from build123d import *

# Parameters (mm, degrees)
CROQUIS1_W              = 29
CROQUIS1_H              = 16
CROQUIS1_R              = 1.5
SALIENTE_EXTRUIR1_DEPTH = 2
CROQUIS2_W              = 3
CROQUIS2_H              = 16
SALIENTE_EXTRUIR2_DEPTH = 17
CROQUIS3_R              = 1.3
CORTAR_EXTRUIR1_DEPTH   = 17
CROQUIS4_W              = 4.8184681
CROQUIS4_H              = 12.262383564
CORTAR_EXTRUIR2_DEPTH   = 10


with BuildPart() as part:
    # Croquis1 → Saliente-Extruir1 (new body)
    with BuildSketch(Plane(origin=(0, 0, 0), x_dir=(1, 0, 0), z_dir=(0, 1, 0))):
        Rectangle(CROQUIS1_W, CROQUIS1_H)
        with Locations(Location((11.5, 0, 0), (0, 0, 270))):
            Circle(CROQUIS1_R, mode=Mode.SUBTRACT)
        with Locations(Location((-11.5, 0, 0), (0, 0, 90))):
            Circle(CROQUIS1_R, mode=Mode.SUBTRACT)
    extrude(amount=SALIENTE_EXTRUIR1_DEPTH)

    # Croquis2 → Saliente-Extruir2 (add)
    with BuildSketch(Plane(origin=(0, 2, 0), x_dir=(1, 0, 0), z_dir=(0, 1, 0))):
        with Locations((4.75, 0)):
            Rectangle(CROQUIS2_W, CROQUIS2_H)
        with Locations((-4.75, 0)):
            Rectangle(CROQUIS2_W, CROQUIS2_H)
    extrude(amount=SALIENTE_EXTRUIR2_DEPTH)

    # Croquis3 → Cortar-Extruir1 (cut)
    with BuildSketch(Plane(origin=(6.25, 0, 0), x_dir=(0, 0, -1), z_dir=(1, 0, 0))):
        with Locations((-4.7, 11.829714682)):
            Circle(CROQUIS3_R)
        with Locations((4.7, 11.829714682)):
            Circle(CROQUIS3_R)
    extrude(amount=-CORTAR_EXTRUIR1_DEPTH, mode=Mode.SUBTRACT)

    # Croquis4 → Cortar-Extruir2 (cut)
    with BuildSketch(Plane(origin=(0, 2, 0), x_dir=(1, 0, 0), z_dir=(0, 1, 0))):
        Rectangle(CROQUIS4_W, CROQUIS4_H)
    extrude(amount=-CORTAR_EXTRUIR2_DEPTH, mode=Mode.SUBTRACT)


solid = part.part
Here's how the part is built. I have some questions about the finished solid (model axes, mm). A direction names the side the tool comes from. Round coordinates to 2 decimals unless told otherwise and drop trailing zeros. Loops run counter-clockwise (first coordinate to the right, second up) from the corner with the lowest first, then second, coordinate; pieces in that order, holes last. Notation, with made-up numbers: (-4.5, 9.5) - (15.5, 9.5) arc R24 cw to (15.5, 34.5) - close; hole circle Ø1 at (16.5, 71). An arc over 180 degrees is marked (long way). One line per question, with ' | ' between items. Start each with the question number.
Q1. Will these pins go through, and if not, where does the flat tip stop? pin 1 (3.5 mm diameter, centred on y = 11.83, z = 4.7, fed in from -X); pin 2 (6 mm diameter, centred on x = 7, z = 5.5, fed in from -Y); pin 3 (8 mm diameter, centred on y = 13.5, z = -1.5, fed in from +X); pin 4 (5 mm diameter, centred on x = 9.5, z = 1.5, fed in from +Y).
Q2. Please list where these lines run through material, in increasing order: line 1 (X direction, y = 1.3, z = 0); line 2 (X direction, y = 8.25, z = -2); line 3 (Z direction, x = 6, y = 11.5). Write a range as [from, to].
Q3. We'd pull the mould along Z, two halves only. Please class faces 1 (the cylindrical face through (-11.95, 0.99, -1.43)), 2 (the flat face through (-4, 7, 8)), 3 (the flat face through (6.25, 10, 0)): +Z half, -Z half, draft (parallel to the pull), parting line (faces both ways), or undercut.
Q4. I want a section at B-B (x = -1). Write out the boundary of the cut face in (y, z).
Q5. I want a section at D-D (z = 6.75). Write out the boundary of the cut face in (x, y).
Q6. I want a section at A-A (z = 0). Write out the boundary of the cut face in (x, y), then the cut area to 3 significant figures.
Q7. For faces 4 (the flat face through (0, 1, -6.131)), 5 (the flat face through (9, 2, 0)), 6 (the flat face through (3.25, 10, 0)), which set-ups out of +Z, -Z, +X, -X, +Y, -Y let a thin tool reach every point of the face, with its end or its side?
Q8. I want a section at C-C (y = 17.5). Write out the boundary of the cut face in (x, z).
Response values:
1) pin 1: stops at x = -6.25 | pin 2: stops at y = 0 | pin 3: stops at x = 6.25 | pin 4: stops at y = 2
2) line 1: x = [-14.5, -13], [-10, -2.41], [2.41, 10], [13, 14.5] | line 2: x = [-6.25, -3.25], [3.25, 6.25] | line 3: z = [-8, -5.96], [-3.44, 3.44], [5.96, 8]
3) face 1: undercut | face 2: +Z half | face 3: draft
4) outline: (0, -8) - (2, -8) - (2, -6.13) - (0, -6.13) - close; (0, 6.13) - (2, 6.13) - (2, 8) - (0, 8) - close
5) outline: (-14.5, 0) - (14.5, 0) - (14.5, 2) - (6.25, 2) - (6.25, 19) - (3.25, 19) - (3.25, 2) - (-3.25, 2) - (-3.25, 19) - (-6.25, 19) - (-6.25, 2) - (-14.5, 2) - close
6) outline: (-14.5, 0) - (-13, 0) - (-13, 2) - (-14.5, 2) - close; (-10, 0) - (-2.41, 0) - (-2.41, 2) - (-3.25, 2) - (-3.25, 19) - (-6.25, 19) - (-6.25, 2) - (-10, 2) - close; (2.41, 0) - (10, 0) - (10, 2) - (6.25, 2) - (6.25, 19) - (3.25, 19) - (3.25, 2) - (2.41, 2) - close; (13, 0) - (14.5, 0) - (14.5, 2) - (13, 2) - close | area: 138 mm²
7) face 4: +Y, -Y | face 5: +Z, -Z, +X, +Y | face 6: +Z, -Z, +Y
8) outline: (-6.25, -8) - (-3.25, -8) - (-3.25, 8) - (-6.25, 8) - close; (3.25, -8) - (6.25, -8) - (6.25, 8) - (3.25, 8) - close
